Autodesk Inventor part; units mm, degrees
ref_plane "YZ Plane" through (0, 0, 0) normal (1, 0, 0) x (0, 1, 0)
ref_plane "XZ Plane" through (0, 0, 0) normal (0, 1, 0) x (-1, 0, 0)
ref_plane "XY Plane" through (0, 0, 0) normal (0, 0, 1) x (1, 0, 0)
sketch "Skizze1" plane through (0, 0, 0) normal (0, 0, 1) x (1, 0, 0)
  line L0 (-9, -18) -> (9, -18)
  line L1 (9, -18) -> (9, 18)
  line L2 (9, 18) -> (-9, 18)
  line L3 (-9, 18) -> (-9, -18)
  line L4 (-9, -18) -> (9, 18) construction
  line L5 (9, -18) -> (-9, 18) construction
  point P0 (0, 0)
  dimension "d0" = 18
  dimension "d1" = 36
extrude "Extrusion1" add sketch "Skizze1" along normal blind 1.2
sketch "Skizze5" plane through (0, 0, 1.2) normal (0, 0, 1) x (1, 0, 0)
  line L0 (4, -13.5) -> (-4, -13.5)
  line L1 (-4, -13.5) -> (-4, -19.5)
  line L2 (-4, -19.5) -> (4, -19.5)
  line L3 (4, -19.5) -> (4, -13.5)
  line L4 (4, -13.5) -> (-4, -19.5) construction
  line L5 (-4, -13.5) -> (4, -19.5) construction
  line L6 (-9, -18) -> (9, -18)
  point P0 (0, 0)
  point P1 (0, -16.5)
  point P2 (0, -16.5)
  dimension "d17" = 8
  dimension "d18" = 6
  dimension "d19" = 4.5
extrude "Extrusion5" add sketch "Skizze5" along normal blind 3
fillet "Rundung1" radius 1.5 4 edges at (4, -16.5, 4.2) (-4, -16.5, 4.2) (-4, -18.75, 1.2) (4, -18.75, 1.2)
sketch "Skizze3" plane through (0, 0, 1.2) normal (0, 0, 1) x (1, 0, 0)
  line L0 (2, 12) -> (-2, 12)
  line L1 (-2, 12) -> (-2, 15)
  line L2 (-2, 15) -> (2, 15)
  line L3 (2, 15) -> (2, 12)
  line L4 (2, 12) -> (-2, 15) construction
  line L5 (-2, 12) -> (2, 15) construction
  line L6 (9, 18) -> (-9, 18)
  point P0 (0, 0)
  point P1 (0, 13.5)
  point P2 (0, 13.5)
  dimension "d8" = 4
  dimension "d9" = 3
  dimension "d10" = 3
extrude "Extrusion3" add sketch "Skizze3" along normal blind 1.2
sketch "Skizze4" plane through (0, 0, 2.4) normal (0, 0, 1) x (1, 0, 0)
  line L0 (-0.5, 13.5) -> (0.5, 13.5) construction
  line L1 (-0.5, 12.9) -> (0.5, 12.9)
  line L2 (0.5, 14.1) -> (-0.5, 14.1)
  arc A0 (-0.5, 14.1) -> (-0.5, 12.9) centre (-0.5, 13.5) ccw
  arc A1 (0.5, 12.9) -> (0.5, 14.1) centre (0.5, 13.5) ccw
  line L3 (-2, 12) -> (2, 12) construction
  line L4 (2, 12) -> (2, 15) construction
  line L5 (2, 15) -> (-2, 15) construction
  line L6 (-2, 15) -> (-2, 12) construction
  line L7 (2, 15) -> (-2, 12) construction
  line L8 (-2, 15) -> (2, 12) construction
  point P0 (0, 0)
  point P1 (0, 13.5)
  point P2 (0, 13.5)
  dimension "d13" = 2.2
  dimension "d14" = 1.2
extrude "Extrusion4" add sketch "Skizze4" along normal blind 1
sketch "Skizze2" plane through (0, 0, 1.2) normal (0, 0, 1) x (1, 0, 0)
  line L0 (5, 0) -> (-5, 0)
  line L1 (-5, 0) -> (-5, 10)
  line L2 (-5, 10) -> (5, 10)
  line L3 (5, 10) -> (5, 0)
  line L4 (5, 0) -> (-5, 10) construction
  line L5 (-5, 0) -> (5, 10) construction
  line L6 (9, 18) -> (-9, 18)
  point P0 (0, 0)
  point P1 (0, 5)
  dimension "d4" = 10
  dimension "d5" = 8
extrude "Extrusion2" add sketch "Skizze2" along normal blind 1.8
properties part number "Teensy"
Here's how the part is built. I have some questions about the finished solid (model axes, mm). A direction names the side the tool comes from. Round coordinates to 2 decimals unless told otherwise and drop trailing zeros. Loops run counter-clockwise (first coordinate to the right, second up) from the corner with the lowest first, then second, coordinate; pieces in that order, holes last. Notation, with made-up numbers: M -28.5,19.25 L -19.5,19.25 A30 cw -19.5,52.25 Z; hole C 12,11 d11. An arc over 180 degrees is marked long. Write each question's results on one line, items separated by ' | '. Start each with the question number.
(1) I want a section at C-C (x = 5.5). Please give me the cut outline in (y, z).
(2) I want a section at B-B (y = 13.5). Please give me the cut outline in (x, z).
(3) I want a section at A-A (z = 1.9). Please give me the cut outline in (x, y).
(4) On a 3-axis mill with a long thin cutter (end or side, diameter ignored), from which of +Z, -Z, +X, -X, +Y, -Y can I reach the whole of each face in a straight line? I mean faces 1 (the flat face through (-5, 5, 2)), 2 (the flat face through (5, 5, 2)), 3 (the flat face through (0, 13.5, 3.4)), 4 (the cylindrical face through (1.1, 13.5, 2.9)). Say none if no direction works.
(5) Thinking about a two-plate mould opening in Y: for faces 5 (the flat face through (0, 12.9, 3)), 6 (the flat face through (0, -16, 4.2)), 7 (the flat face through (0, -18, 1)), which applies, pulls with the +Y half, pulls with the -Y half, needs draft (parallel to the pull), parting line crosses it, or undercut?
(6) If I drill on probe 1 along Y at (x, z) = (0.75, 1.9); probe 2 along Z at (x, y) = (-3, 6.5); probe 3 along Z at (x, y) = (8.25, -4.5), over which ranges is the centre line in solid material (lowest first)? Write a range as from..to.
(7) Will these pins go through, and if not, where does the flat tip stop? P1, Ø0.5, axis at x = 0, z = 2.5, coming from the +Y side; P2, Ø5, axis at x = 5.5, y = 12, coming from the +Z side; P3, Ø0.6, axis at y = 13.5, z = 2, coming from the -X side.
Solved:
1) outline: M -18,0 L 18,0 L 18,1.2 L -18,1.2 Z
2) outline: M -9,0 L 9,0 L 9,1.2 L 2,1.2 L 2,2.4 L 1.1,2.4 L 1.1,3.4 L -1.1,3.4 L -1.1,2.4 L -2,2.4 L -2,1.2 L -9,1.2 Z
3) outline: M -5,0 L 5,0 L 5,10 L -5,10 Z; M -4,-18 L -3.77,-18 L -3.77,-19.5 L 3.77,-19.5 L 3.77,-18 L 4,-18 L 4,-13.5 L -4,-13.5 Z; M -2,12 L 2,12 L 2,15 L -2,15 Z
4) face 1: +Z, -X, +Y, -Y | face 2: +Z, +X, +Y, -Y | face 3: +Z, +X, -X, +Y | face 4: +Z, +X
5) face 5: undercut | face 6: needs draft | face 7: pulls with the -Y half
6) probe 1: y = -19.5..-13.5, 0..10, 12..15 | probe 2: z = 0..3 | probe 3: z = 0..1.2
7) P1: stops at y = 15 | P2: stops at z = 3 | P3: stops at x = -2
